Drawing for the job (mm, zero at the part's lowest x, y, z). Coordinates: 2 decimals unless noted, no trailing zeros. Order: outer loops, then holes, each group sorted by start corner. A loop starts at its lowest first (then second) coordinate and runs counter-clockwise, first axis right, second up. Notation, with made-up numbers: (24.5, 3) - (47.5, 3) arc R27 cw to (47.5, 23) - close; hole circle Ø1 at (43, -6). An arc over 180 degrees is marked (long way). Put each result on its own line as item: value. Start each with the question number.
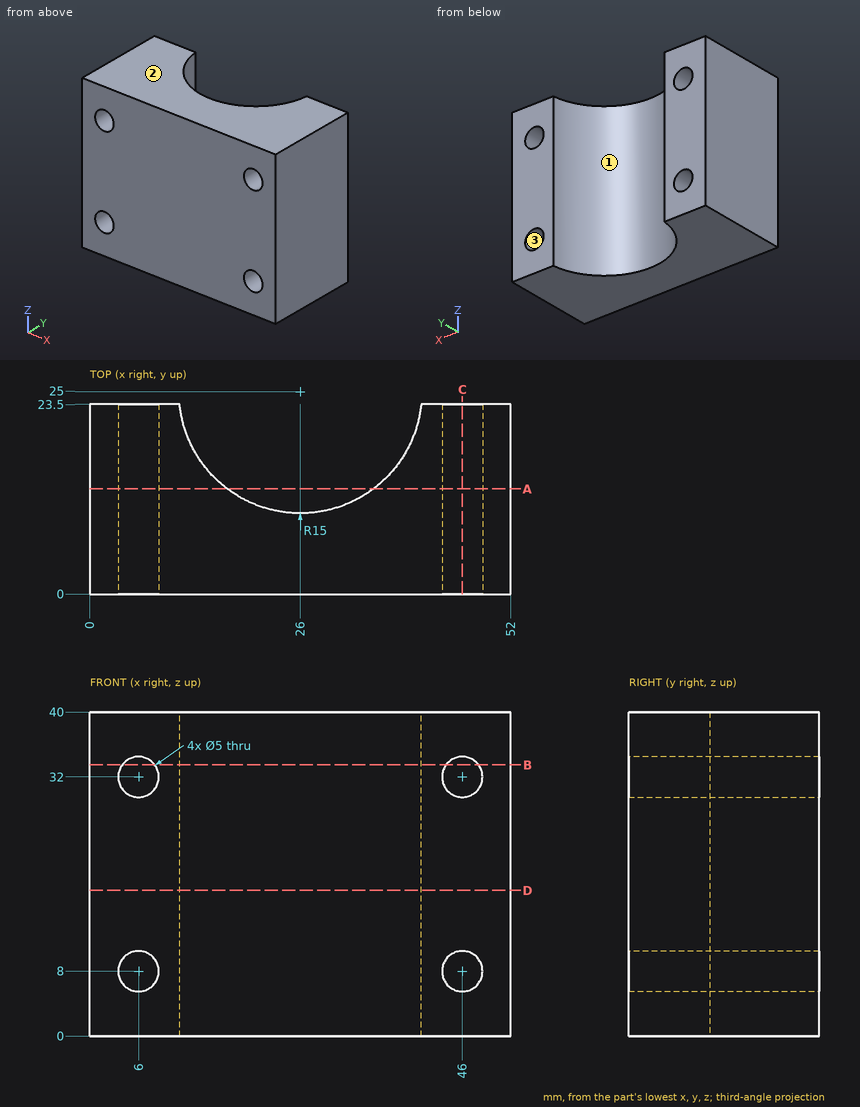
Item 1: Slice it at D-D, the plane z = 18. Give the cut face in (x, y), plus the area to 3 significant figures.
Item 2: Flat gauge pins, fed straight in: pin 1 Ø3 at (x, z) = (6, 32) entering from -Y; pin 2 Ø1.5 at (x, z) = (22.5, 16.5) entering from +Y; pin 3 Ø10 at (x, y) = (39.5, 16.5) entering from -Z; pin 4 Ø5 at (x, z) = (21, 28.5) entering from +Y. Where does each tip first touch, or does it go through?
Item 3: Wall check: line 1 along X through (y, z) = (8.5, 8); line 2 along Z through (x, y) = (7, 18.5); line 3 along Z through (x, y) = (45.5, 5.5). Give the ranges that are in metal, low to high.
Item 4: Slice it at A-A, the plane y = 13. Give the cut face in (x, z), plus the area to 3 significant figures.
Item 5: Slice it at B-B, the plane z = 33.5. Give the cut face in (x, y), plus the area to 3 significant figures.
Item 6: Pull direction Z, two halves, no side cores. Call the marked faces 1, 2 and 3: pulls with the +Z half, pulls with the -Z half, needs draft (parallel to the pull), parting line crosses it, or undercut.
Item 7: Slice it at C-C, the plane x = 46. Give the cut face in (y, z).
Here are the results:
1. outline: (0, 0) - (52, 0) - (52, 23.5) - (40.92, 23.5) arc R15 cw to (11.08, 23.5) - (0, 23.5) - close
1. area: 913 mm^2
2. pin 1: passes through
2. pin 2: stops at y = 10.61
2. pin 3: stops at z = 0
2. pin 4: stops at y = 12.01
3. line 1: x = 0 to 3.5, 8.5 to 43.5, 48.5 to 52
3. line 2: z = 0 to 5.71, 10.29 to 29.71, 34.29 to 40
3. line 3: z = 0 to 5.55, 10.45 to 29.55, 34.45 to 40
4. outline: (0, 0) - (17, 0) - (17, 40) - (0, 40) - close; (35, 0) - (52, 0) - (52, 40) - (35, 40) - close; hole circle Ø5 at (6, 8); hole circle Ø5 at (6, 32); hole circle Ø5 at (46, 8); hole circle Ø5 at (46, 32)
4. area: 1,280 mm^2
5. outline: (0, 0) - (4, 0) - (4, 23.5) - (0, 23.5) - close; (8, 0) - (44, 0) - (44, 23.5) - (40.92, 23.5) arc R15 cw to (11.08, 23.5) - (8, 23.5) - close; (48, 0) - (52, 0) - (52, 23.5) - (48, 23.5) - close
5. area: 725 mm^2
6. face 1: needs draft
6. face 2: pulls with the +Z half
6. face 3: undercut
7. outline: (0, 0) - (23.5, 0) - (23.5, 5.5) - (0, 5.5) - close; (0, 10.5) - (23.5, 10.5) - (23.5, 29.5) - (0, 29.5) - close; (0, 34.5) - (23.5, 34.5) - (23.5, 40) - (0, 40) - close
